Answer from the drawing. Dimensions are ordinates in mm from the lowest x, y and z of the part. A direction names the side the tool comes from. Coordinates: 2 decimals unless noted, no trailing zeros. Write each loop counter-clockwise with the first axis right and the second up, starting at its lowest first coordinate (ties: lowest second). Pieces come first, ordered by that corner, then holes.
(1) Which of the six approach directions +Z, -Z, +X, -X, +Y, -Y give full straight-line access (tool end or side, diameter ignored) to the marked faces 1 and 2?
(2) Section A-A on z = 15 is taken. Write down the section's boundary in (x, y).
(3) Section C-C on z = 4 is taken. Write down the section's boundary in (x, y).
(4) Find the intervals of material crossed by probe 1 along Y at (x, z) = (7.25, 15); probe 2 along Y at (x, z) = (1.25, 25.5) (1 decimal); probe 3 along X at (y, z) = (25.5, 12.5), in increasing order.
(5) Given pin 1 (3 mm diameter, centred on x = 1.5, z = 7, fed in from +Y); pin 2 (6 mm diameter, centred on y = 15.5, z = 8.5, fed in from -X); pin 3 (1.2 mm diameter, centred on y = 26, z = 15, fed in from +X); pin 4 (2 mm diameter, centred on x = 7, z = 7.5, fed in from -Y), each flat-ended and moving along its own axis, determine where each tip first touches the part or whether it passes through.
(6) Section B-B on y = 12 is taken. Write down the section's boundary in (x, z) (1 decimal).
(7) The mould has two halves that part along Y. Classify the marked faces 3, 4, 5 and 6: +Y half, -Y half, draft (parallel to the pull), parting line (faces both ways), or undercut.
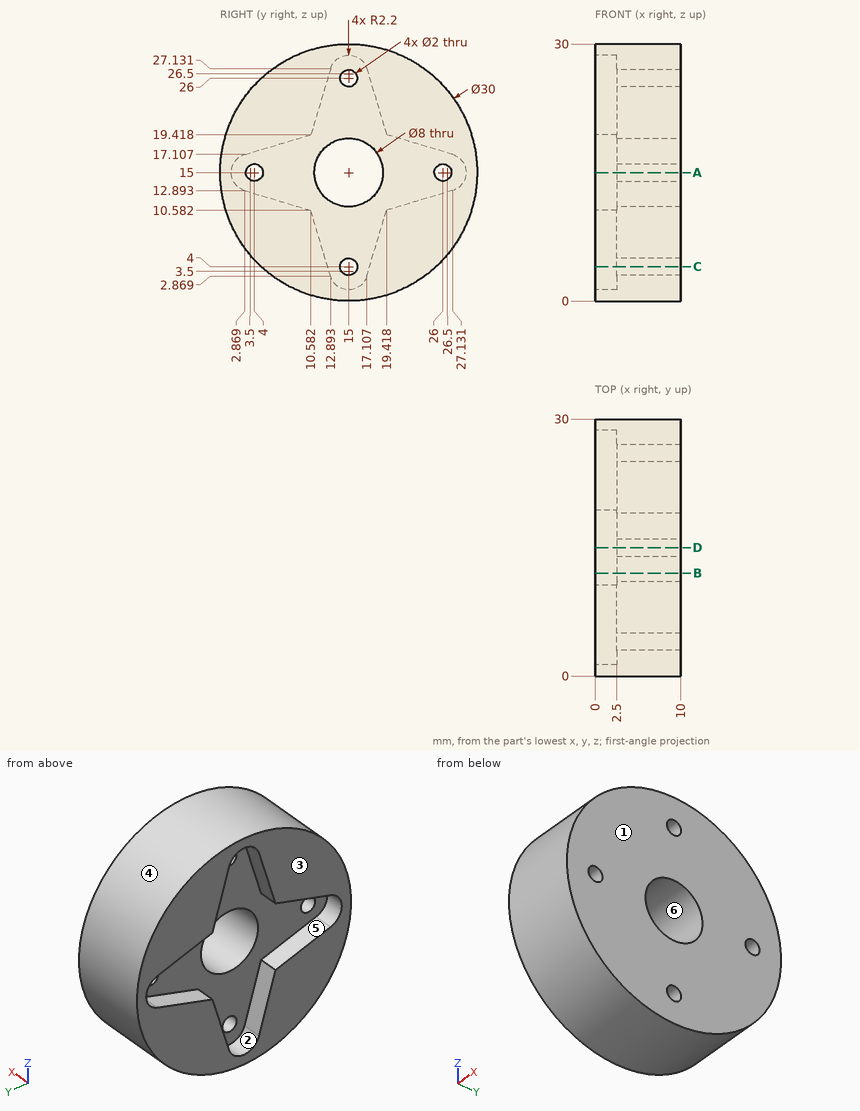
Response:
1. face 1: +Z, -Z, +X, +Y, -Y
1. face 2: -X
2. outline: (0, 0) - (10, 0) - (10, 3) - (2.5, 3) - (2.5, 1.3) - (0, 1.3) - close; (0, 28.7) - (2.5, 28.7) - (2.5, 27) - (10, 27) - (10, 30) - (0, 30) - close; (2.5, 5) - (10, 5) - (10, 11) - (2.5, 11) - close; (2.5, 19) - (10, 19) - (10, 25) - (2.5, 25) - close
3. outline: (0, 4.8) - (10, 4.8) - (10, 14) - (2.5, 14) - (2.5, 12.55) - (0, 12.55) - close; (0, 17.45) - (2.5, 17.45) - (2.5, 16) - (10, 16) - (10, 25.2) - (0, 25.2) - close
4. probe 1: y = 0 to 3, 5 to 11, 19 to 25, 27 to 30
4. probe 2: y = 4.3 to 12.4, 17.6 to 25.7
4. probe 3: x = 2.5 to 10
5. pin 1: stops at y = 28.52
5. pin 2: stops at x = 2.5
5. pin 3: passes through
5. pin 4: stops at y = 1.48
6. outline: (0, 0.3) - (10, 0.3) - (10, 12.4) - (2.5, 12.4) - (2.5, 5.8) - (0, 5.8) - close; (0, 24.2) - (2.5, 24.2) - (2.5, 17.6) - (10, 17.6) - (10, 29.7) - (0, 29.7) - close
7. face 3: draft
7. face 4: parting line
7. face 5: undercut
7. face 6: undercut
